from build123d import *

# Parameters (mm, degrees)
F3_D           = 3.302
F3_DEPTH       = 25.4
F3_CSINK_D     = 7.62
F3_CSINK_ANGLE = 82
F3_TIP         = 0.992020882
F5_DEPTH       = 7.62
F6_R           = 1.016


with BuildPart() as f1:
    # F0 (on Front) → F1 (revolve)
    with BuildSketch(Plane.XZ):
        with BuildLine():
            Line((-3.175, 6.35), (-3.175, 0))
            Line((-3.175, 0), (-19.05, 0))
            Line((-19.05, 0), (-19.05, -5.08))
            Line((-19.05, -5.08), (0, -5.08))
            Line((0, -5.08), (0, 38.1))
            add(Edge.make_bspline(
                [(-3.175, 6.35), (-7.2207896582, 6.2912448099), (-10.1526060146, 9.7732957635), (-12.0009457177, 18.875299473), (-4.072510735, 38.1), (0, 38.1)],
                knots=[0, 0, 0, 0, 0.2584564677, 0.5593342036, 1, 1, 1, 1], degree=3))
        make_face()
    revolve(axis=Axis((0, 0, 12.1911335737), (0, 0, -1)))

    # F3
    with Locations(Plane(origin=(0, 0, -5.08), x_dir=(1, 0, 0), z_dir=(0, 0, -1))):
        with Locations((0, 0)):
            CounterSinkHole(F3_D / 2, F3_CSINK_D / 2, depth=F3_DEPTH, counter_sink_angle=F3_CSINK_ANGLE)
            with Locations((0, 0, -(F3_DEPTH + F3_TIP / 2))):  # 118° drill point
                Cone(0, F3_D / 2, F3_TIP, mode=Mode.SUBTRACT)

    # F4 (on face) → F5 (cut)
    with BuildSketch(Plane(origin=(0, 0, -5.08), x_dir=(1, 0, 0), z_dir=(0, 0, -1))):
        with BuildLine():
            Line((-6.604, -17.8686788544), (-6.604, 17.8686788544))
            ThreePointArc((-6.604, 17.8686788544), (-19.05, 0), (-6.604, -17.8686788544))
        make_face()
        with BuildLine():
            ThreePointArc((19.05, 0), (15.6318377039, 10.8879819067), (6.604, 17.8686788544))
            Line((6.604, 17.8686788544), (6.604, -17.8686788544))
            ThreePointArc((6.604, -17.8686788544), (15.6318377039, -10.8879819067), (19.05, 0))
        make_face()
    extrude(amount=-F5_DEPTH, mode=Mode.SUBTRACT)

    # F6
    f6_edges = [f1.edges().sort_by_distance(p)[0] for p in [
        (3.175, 0, 6.35),
        (3.175, 0, 0),
        (0, 19.05, 0),
        (0, 19.05, -5.08),
        (-6.604, 0, -5.08),
        (6.604, 0, -5.08),
        (-6.604, 0, 0),
        (6.604, 0, 0),
        (6.604, -17.868679, -2.54),
        (6.604, 17.868679, -2.54),
        (-6.604, -17.868679, -2.54),
        (-6.604, 17.868679, -2.54),
        (0, -19.05, 0),
        (0, -19.05, -5.08),
    ]]
    fillet(f6_edges, radius=F6_R)


solid = f1.part
CAD build for the part. Positions are in the model's coordinates, mm. A direction names the side the tool comes from. Coordinates: 2 decimals unless noted, no trailing zeros. Order: outer loops, then holes, each group sorted by start corner. A loop starts at its lowest first (then second) coordinate and runs counter-clockwise, first axis right, second up.
Item 1: Two-plate mould, pull along Z, no slides. Class faces 1 (the face through (6.314, 0.24, -4.774)), 2 (the face through (6.405, 17.75, -2.519)), 3 (the face through (-6.3, 0.24, -0.29)): +Z half, -Z half, draft (parallel to the pull), parting line (faces both ways), or undercut.
Check sheet entries:
face 1: -Z half
face 2: draft
face 3: undercut
Item 2: Drill centre lines: L1, parallel to Z at x = -1.25, y = -11; L2, parallel to Z at x = 5.5, y = -5.5; L3, parallel to Y at x = 0, z = 13.5. Where is each one in solid material? Low to high.
Check sheet entries:
L1: z = -5.08 to 0
L2: z = -5.08 to 0, 7.54 to 27.7
L3: y = -10.61 to -1.65, 1.65 to 10.61
Item 3: Band-saw the part on A-A on y = 12.5. List the corners of the cut face in (x, z).
Check sheet entries:
outline: (-6.6, -4.06) arc R1.02 ccw to (-5.59, -5.08) - (5.59, -5.08) arc R1.02 ccw to (6.6, -4.06) - (6.6, -1.02) arc R1.02 ccw to (5.59, 0) - (-5.59, 0) arc R1.02 ccw to (-6.6, -1.02) - close
Item 4: Band-saw the part on B-B on z = 4.5. List the corners of the cut face in (x, y) (3 decimals), plus the area to 3 significant figures.
Check sheet entries:
outline: circle Ø6.35 at (0, 0); hole circle Ø3.302 at (0, 0)
area: 23.1 mm2
Item 5: Pin check, flat tips, straight feed: pin 1 Ø3 at (x, z) = (-7.5, 10.5) entering from -Y; pin 2 Ø1.5 at (x, z) = (4, 3) entering from -Y; pin 3 Ø1.5 at (y, z) = (8, -2.5) entering from -X; pin 4 Ø12 at (x, z) = (3.5, 2.5) entering from +Y. Stop position of each tip, or through.
Check sheet entries:
pin 1: stops at y = -7.98
pin 2: passes through
pin 3: stops at x = -6.6
pin 4: stops at y = 19.05
Item 6: 3-axis set-ups, long thin cutter, end or side, ignore diameter. For faces 4 (the face through (-6.604, 0, -3)), 5 (the face through (-2.93, -1.22, 3.16)), 6 (the face through (6.604, 0, -3)), 7 (the face through (6.3, -0.24, -0.29)), 8 (the face through (-1.525, 0.632, 9.022)): which of +Z, -Z, +X, -X, +Y, -Y reach the whole face in a straight line?
Check sheet entries:
face 4: -Z, -X, +Y, -Y
face 5: none
face 6: -Z, +X, +Y, -Y
face 7: +X, +Y, -Y
face 8: -Z
